Can you work these out from the drawing? Everything is in mm from the part's minimum corner. A direction names the side the tool comes from. Coordinates: 2 decimals unless noted, no trailing zeros. Order: outer loops, then holes, each group sorted by start corner. A loop starts at its lowest first (then second) coordinate and runs counter-clockwise, first axis right, second up. Notation, with made-up numbers: (7.5, -38) - (46.5, -38) arc R10 cw to (46.5, -19) - close; hole circle Ø5 at (44.25, -34). An arc over 180 degrees is marked (long way). Use a Markdown table: item, result. Add a question column.
(1) For pin 1 Ø10 at (y, z) = (26, 21.5) entering from +X (3 decimals); pin 2 Ø6.5 at (y, z) = (13, 19) entering from -X (3 decimals); pin 3 Ø4.5 at (x, y) = (76.2, 22.225) entering from +Z; pin 4 Ø10 at (x, z) = (43, 19) entering from -Y (3 decimals), each with a flat end and sliding along its axis, tell me the tip position at first contact or that it passes through.
(2) I want a section at B-B (y = 6). List the corners of the cut face in (x, z) for me (1 decimal), and give its area (3 significant figures).
(3) I want a section at C-C (z = 23). List the corners of the cut face in (x, y) for me (1 decimal), and give its area (3 significant figures).
(4) If I drill on L1, parallel to X at y = 23.5, z = 8; L2, parallel to X at y = 20.5, z = 12 (1 decimal); L3, parallel to Y at x = 80, z = 24 (1 decimal), over which ranges is the centre line in solid material (lowest first)? Write a range as [from, to].
(5) On a 3-axis mill with a long thin cutter (end or side, diameter ignored), from which of +Z, -Z, +X, -X, +Y, -Y can I reach the whole of each face in a straight line? I mean the marked faces 1, 2 and 3. Say none if no direction works.
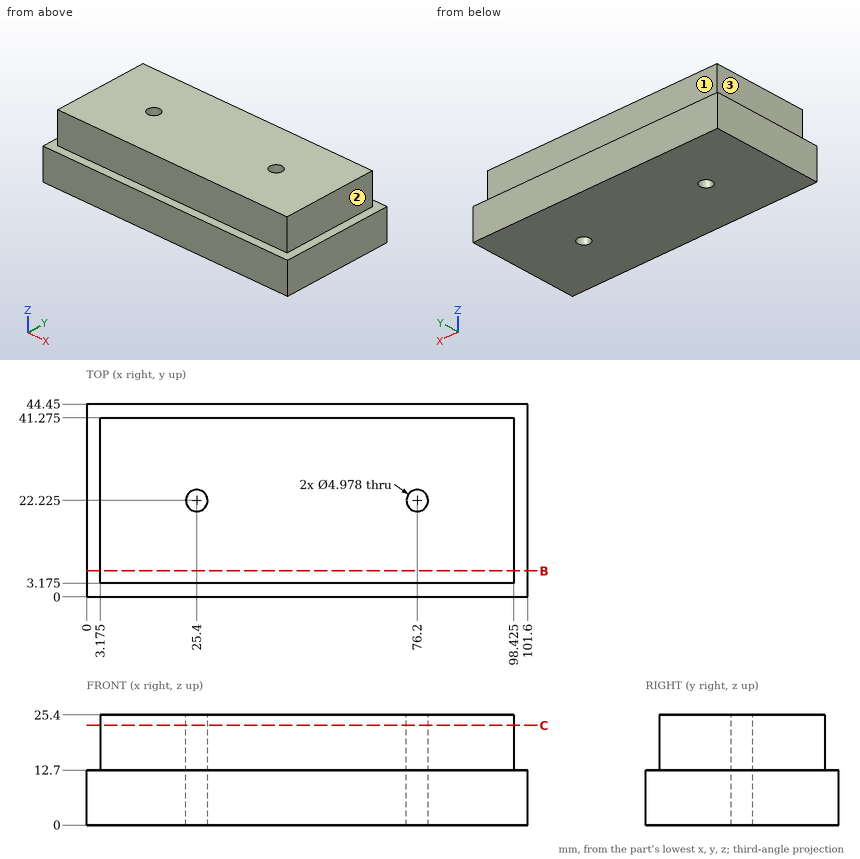
Answers follow:
| question | item | result |
|---|---|---|
| 1 | pin 1 | stops at x = 98.425 |
| 1 | pin 2 | stops at x = 3.175 |
| 1 | pin 3 | passes through |
| 1 | pin 4 | stops at y = 3.175 |
| 2 | outline | (0, 0) - (101.6, 0) - (101.6, 12.7) - (98.4, 12.7) - (98.4, 25.4) - (3.2, 25.4) - (3.2, 12.7) - (0, 12.7) - close |
| 2 | area | 2,500 mm² |
| 3 | outline | (3.2, 3.2) - (98.4, 3.2) - (98.4, 41.3) - (3.2, 41.3) - close; hole circle Ø5 at (25.4, 22.2); hole circle Ø5 at (76.2, 22.2) |
| 3 | area | 3,590 mm² |
| 4 | L1 | x = [0, 23.26], [27.54, 74.06], [78.34, 101.6] |
| 4 | L2 | x = [0, 23.6], [27.2, 74.4], [78, 101.6] |
| 4 | L3 | y = [3.2, 41.3] |
| 5 | face 1 | +Z, +X, -X, +Y |
| 5 | face 2 | +Z, +X, +Y, -Y |
| 5 | face 3 | +Z, -X, +Y, -Y |
